from build123d import *

# Parameters (mm, degrees)
SKETCH1_R           = 1.5
SKETCH1_R_2         = 1.435
SKETCH1_R_3         = 3
BOSS_EXTRUDE1_DEPTH = 3.175


with BuildPart() as part:
    # Sketch1 → Boss-Extrude1 (new body)
    with BuildSketch(Plane.XY):
        Polygon((3.175, 0), (3.175, -3.175), (9.525, -3.175), (9.525, 0), (15.875, 0), (15.875, -3.175), (22.225, -3.175), (22.225, 0), (79.375, 0), (79.375, -3.175), (85.725, -3.175), (85.725, 0), (92.075, 0), (92.075, -3.175), (98.425, -3.175), (98.425, 0), (101.6, 0), (101.6, 36.195), (98.425, 36.195), (98.425, 39.37), (92.075, 39.37), (92.075, 36.195), (85.725, 36.195), (85.725, 39.37), (79.375, 39.37), (79.375, 36.195), (22.225, 36.195), (22.225, 39.37), (15.875, 39.37), (15.875, 36.195), (9.525, 36.195), (9.525, 39.37), (3.175, 39.37), (3.175, 36.195), (0, 36.195), (0, 0), align=None)
        with Locations((34.585, 5)):
            Circle(SKETCH1_R, mode=Mode.SUBTRACT)
        with Locations((27.7875, 5)):
            Circle(SKETCH1_R_2, mode=Mode.SUBTRACT)
        with Locations(Location((67.015, 5, 0), (0, 0, 180))):
            Circle(SKETCH1_R, mode=Mode.SUBTRACT)
        with Locations(Location((73.8125, 5, 0), (0, 0, 180))):
            Circle(SKETCH1_R_2, mode=Mode.SUBTRACT)
        with Locations((50.8, 5)):
            Circle(SKETCH1_R_3, mode=Mode.SUBTRACT)
    extrude(amount=BOSS_EXTRUDE1_DEPTH)


solid = part.part
CAD build for the part. Positions are in the model's coordinates, mm. A direction names the side the tool comes from. Round coordinates to 2 decimals unless told otherwise and drop trailing zeros. Loops run counter-clockwise (first coordinate to the right, second up) from the corner with the lowest first, then second, coordinate; pieces in that order, holes last. Notation, with made-up numbers: M 22.25,15.25 L 46.25,15.25 A10 ccw 46.25,24.25 Z; hole C -7,-39 d8. An arc over 180 degrees is marked long. One line per question, with ' | ' between items. Start each with the question number.
Item 1: Cut at D-D, the plane x = 50.8. Write the cut outline in (y, z) (3 decimals).
Item 2: Cut at B-B, the plane x = 28. Write the cut outline in (y, z) (3 decimals).
Item 3: Wall check: line 1 (X direction, y = -0.5, z = 0.2) (3 decimals); line 2 (Y direction, x = 50.8, z = 0.8) (3 decimals); line 3 (Y direction, x = 46, z = 3) (3 decimals). Give the ranges that are in metal, low to high.
Item 4: Which spindle directions (+Z, -Z, +X, -X, +Y, -Y) get a long thin tool onto all of the face, cutting with end or side? Do faces 1 (the flat face through (92.075, -2, 2)), 2 (the flat face through (50, 18, 3.175)), 3 (the flat face through (2, 36.195, 2)), 4 (the flat face through (2, 0, 2)), 5 (the flat face through (22.225, 38, 2)). Say none if no direction does.
Item 5: Pin check, flat tips, straight feed: pin 1 Ø1 at (x, z) = (28.5, 2) entering from -Y; pin 2 Ø1.6 at (y, z) = (37.5, 1.5) entering from -X (3 decimals); pin 3 Ø1 at (x, z) = (37.5, 1) entering from +Y (3 decimals). Stop position of each tip, or through.
Item 6: Two-plate mould, pull along X, no slides. Class faces 6 (the cylindrical face through (68.514, 4.934, 1.565)), 7 (the flat face through (22.225, -2, 2)), 8 (the flat face through (83, 39.37, 2)), 9 (the flat face through (3.175, -2, 2)): pulls with the +X half, pulls with the -X half, needs draft (parallel to the pull), parting line crosses it, or undercut.
Item 7: Cut at C-C, the plane z = 1.7. State how many separate pieces and enclosed holes the cut face has, plus the area to 3 significant figures.
Item 8: Cut at A-A, the plane y = 5. Write the cut outline in (x, z) (1 decimal), plus the area to 3 significant figures.
Responses:
1) outline: M 0,0 L 2,0 L 2,3.175 L 0,3.175 Z; M 8,0 L 36.195,0 L 36.195,3.175 L 8,3.175 Z
2) outline: M 0,0 L 3.581,0 L 3.581,3.175 L 0,3.175 Z; M 6.419,0 L 36.195,0 L 36.195,3.175 L 6.419,3.175 Z
3) line 1: x = 3.175 to 9.525, 15.875 to 22.225, 79.375 to 85.725, 92.075 to 98.425 | line 2: y = 0 to 2, 8 to 36.195 | line 3: y = 0 to 36.195
4) face 1: +Z, -Z, -Y | face 2: +Z, +X, -X, +Y, -Y | face 3: +Z, -Z, -X, +Y | face 4: +Z, -Z, -X, -Y | face 5: +Z, -Z, +Y
5) pin 1: stops at y = 0 | pin 2: stops at x = 3.175 | pin 3: stops at y = 36.195
6) face 6: undercut | face 7: undercut | face 8: needs draft | face 9: pulls with the -X half
7) separate pieces: 1 | enclosed holes: 5 | area: 3,780 mm²
8) outline: M 0,0 L 26.4,0 L 26.4,3.2 L 0,3.2 Z; M 29.2,0 L 33.1,0 L 33.1,3.2 L 29.2,3.2 Z; M 36.1,0 L 47.8,0 L 47.8,3.2 L 36.1,3.2 Z; M 53.8,0 L 65.5,0 L 65.5,3.2 L 53.8,3.2 Z; M 68.5,0 L 72.4,0 L 72.4,3.2 L 68.5,3.2 Z; M 75.2,0 L 101.6,0 L 101.6,3.2 L 75.2,3.2 Z | area: 266 mm²
